```python
from build123d import *

# Parameters (mm, degrees)
F1_DEPTH  = 25
F2_R      = 1.75
F3_DEPTH  = 12.001
F4_W      = 2.25
F4_H      = 5.2
F5_DEPTH  = 8.2
F6_W      = 6.7676874548
F6_H      = 2
F6_W_2    = 4.3625808284
F6_H_2    = 16.5741704404
F7_DEPTH  = 25.001
F8_R      = 1.1
F9_DEPTH  = 11
F10_W     = 7.5431205352
F10_H     = 29.8151662209
F11_DEPTH = 12


with BuildPart() as f1:
    # F0 (on Top) → F1 (new body)
    with BuildSketch(Plane.XY):
        Polygon((11.3658751324, 15), (7.8658751324, 15), (7.8658751324, -17), (19.8658751324, -17), (19.8658751324, 15), (14.9658751324, 15), (14.9658751324, 0), (11.3658751324, 0), align=None)
    extrude(amount=F1_DEPTH)

    # F2 (on face) → F3 (cut, through all)
    with BuildSketch(Plane(origin=(7.8658751324, 0, 0), x_dir=(0, -1, 0), z_dir=(-1, 0, 0))):
        with Locations((-10, 17)):
            Circle(F2_R)
        with Locations((-10, 7)):
            Circle(F2_R)
    extrude(amount=-F3_DEPTH, mode=Mode.SUBTRACT)

    # F4 (on face) → F5 (cut)
    with BuildSketch(Plane(origin=(0, 15, 0), x_dir=(-1, 0, 0), z_dir=(0, 1, 0))):
        with Locations((-17.2876401603, 17)):
            Rectangle(F4_W, F4_H)
        with Locations((-17.2876401603, 6.9)):
            Rectangle(F4_W, F4_H)
    extrude(amount=-F5_DEPTH, mode=Mode.SUBTRACT)

    # F6 (on face) → F7 (cut, through all)
    with BuildSketch(Plane.XY.offset(25)):
        with Locations((17.0719223097, 14.3433604389)):
            Rectangle(F6_W, F6_H)
        with Locations((9.1845847182, 8.2870852202)):
            Rectangle(F6_W_2, F6_H_2)
    extrude(amount=-F7_DEPTH, mode=Mode.SUBTRACT)

    # F8 (on face) → F9 (cut)
    with BuildSketch(Plane(origin=(7.8658751324, 0, 0), x_dir=(0, -1, 0), z_dir=(-1, 0, 0))):
        Polygon((16.5, 22.9742758833), (0.5, 22.9742758833), (0.5, 2.4742758833), (16.5, 2.4742758833), (16.5, 11.9742758833), (19.0740358084, 11.9742758833), (19.0740358084, 22.9742758833), align=None)
        with Locations((8.5, 7.4742758833)):
            Circle(F8_R, mode=Mode.SUBTRACT)
        with Locations((8.5, 17.4742758833)):
            Circle(F8_R, mode=Mode.SUBTRACT)
    extrude(amount=-F9_DEPTH, mode=Mode.SUBTRACT)

    # F10 (on face) → F11 (cut)
    with BuildSketch(Plane.XZ.offset(17)):
        with Locations((9.0943148648, 13.0673133535)):
            Rectangle(F10_W, F10_H)
    extrude(amount=-F11_DEPTH, mode=Mode.SUBTRACT)


solid = f1.part
```
Design review of the part built by this model. Coordinates are the model's own, in mm. A direction names the side the tool comes from. Coordinates: 2 decimals unless noted, no trailing zeros. Order: outer loops, then holes, each group sorted by start corner. A loop starts at its lowest first (then second) coordinate and runs counter-clockwise, first axis right, second up. Notation, with made-up numbers: (2.5, 18.25) - (17.5, 18.25) arc R23 cw to (17.5, 55.25) - close; hole circle Ø9 at (7, 50). An arc over 180 degrees is marked (long way). One line per question, with ' | ' between items.
Q1. Consider section A-A, the plane y = 10. Give the boundary of the cut face in (x, z), then the cut area to 4 significant figures.
Answer key:
outline: (14.97, 0) - (19.87, 0) - (19.87, 5.25) - (18.41, 5.25) - (18.41, 4.3) - (16.16, 4.3) - (16.16, 5.25) - (14.97, 5.25) - close; (14.97, 8.75) - (16.16, 8.75) - (16.16, 9.5) - (18.41, 9.5) - (18.41, 8.75) - (19.87, 8.75) - (19.87, 15.25) - (18.41, 15.25) - (18.41, 14.4) - (16.16, 14.4) - (16.16, 15.25) - (14.97, 15.25) - close; (14.97, 18.75) - (16.16, 18.75) - (16.16, 19.6) - (18.41, 19.6) - (18.41, 18.75) - (19.87, 18.75) - (19.87, 25) - (14.97, 25) - close | area: 80.55 mm2
Q2. To check wall thickness, follow line 1 along Z through (x, y) = (18.8, 10); line 2 along Z through (x, y) = (17.5, 7.5); line 3 along Z through (x, y) = (16, -13.5). State the ranges of each line that lie inside material, in increasing order.
Answer key:
line 1: z = 0 to 5.25, 8.75 to 15.25, 18.75 to 25 | line 2: z = 0 to 4.3, 9.5 to 14.4, 19.6 to 25 | line 3: z = 0 to 2.47, 22.97 to 25
Q3. Consider section B-B, the plane x = 17.25. Give the boundary of the cut face in (y, z), then the cut area to 3 significant figures.
Answer key:
outline: (-17, 0) - (13.34, 0) - (13.34, 4.3) - (6.8, 4.3) - (6.8, 9.5) - (13.34, 9.5) - (13.34, 14.4) - (6.8, 14.4) - (6.8, 19.6) - (13.34, 19.6) - (13.34, 25) - (-17, 25) - (-17, 22.97) - (-0.5, 22.97) - (-0.5, 2.47) - (-16.5, 2.47) - (-16.5, 11.97) - (-17, 11.97) - close; circle Ø2.2 at (-8.5, 7.47); circle Ø2.2 at (-8.5, 17.47) | area: 365 mm2
Q4. The part is to be moulded in two halves that separate along Z. For faces 5 (the flat face through (10, -5, 24)), 6 (the flat face through (18.413, 10, 5)), 7 (the flat face through (15, -2, 25)), say which applies: +Z half, -Z half, draft (parallel to the pull), parting line (faces both ways), or undercut.
Answer key:
face 5: draft | face 6: undercut | face 7: +Z half
Q5. Consider section D-D, the plane x = 11.25. Give the boundary of the cut face in (y, z), then the cut area to 4 significant figures.
Answer key:
outline: (-5, 0) - (0, 0) - (0, 25) - (-5, 25) - (-5, 22.97) - (-0.5, 22.97) - (-0.5, 2.47) - (-5, 2.47) - close | area: 32.75 mm2
Q6. Consider section C-C, the plane z = 17. Give the boundary of the cut face in (x, y), then the cut area to 3 significant figures.
Answer key:
outline: (7.87, -0.5) - (18.87, -0.5) - (18.87, -7.51) - (12.87, -7.51) - (12.87, -9.49) - (18.87, -9.49) - (18.87, -17) - (19.87, -17) - (19.87, 8.25) - (18.41, 8.25) - (18.41, 6.8) - (16.16, 6.8) - (16.16, 8.25) - (14.97, 8.25) - (14.97, 0) - (7.87, 0) - close; (14.97, 11.75) - (16.16, 11.75) - (16.16, 13.34) - (14.97, 13.34) - close; (18.41, 11.75) - (19.87, 11.75) - (19.87, 13.34) - (18.41, 13.34) - close | area: 75.8 mm2
Q7. Clearance check with flat-ended pins moving along their axes: pin 1 Ø4 at (y, z) = (9.5, 18.5) entering from -X; pin 2 Ø1.8 at (y, z) = (-9, 8) entering from -X; pin 3 Ø3 at (x, z) = (13, 19.5) entering from +Y. State where each tip first meets the part, or that it passes through.
Answer key:
pin 1: stops at x = 14.97 | pin 2: stops at x = 12.87 | pin 3: stops at y = 0
Q8. For faces 1 (the flat face through (12.866, -11, 2)), 2 (the cylindrical face through (19.129, 10.228, 18.735)), 3 (the flat face through (16.163, 10, 5)), 4 (the cylindrical face through (15.824, -8.357, 18.565)), list the 3-axis set-ups (+Z, -Z, +X, -X, +Y, -Y) from which the entire face can be reached by the end or side of a thin tool; tool diameter is ignored.
Answer key:
face 1: +Z, -Z, -X, -Y | face 2: +X, -X | face 3: +Y | face 4: -X
